Geometry: final body of the model. Coordinates: model frame, mm. A direction names the side the tool comes from. Give positions to 0.01 mm unless a question says otherwise; leave off trailing zeros. Loops run counter-clockwise (first coordinate to the right, second up) from the corner with the lowest first, then second, coordinate; pieces in that order, holes last. Notation, with made-up numbers: (-13.75, 0.25) -> (40.25, 0.25) arc R18 cw to (40.25, 17.25) -> close; hole circle Ø4 at (50.25, -21). An arc over 180 degrees is marked (long way). Answer in a Markdown table with one row per item. Add a question column.
from build123d import *

# Parameters (mm, degrees)
SKETCH1_W           = 80
SKETCH1_H           = 40
SKETCH1_R           = 1.5
SKETCH1_R_2         = 3
BOSS_EXTRUDE1_DEPTH = 4
EDGE_FLANGE1_DEPTH  = 40
SKETCH13_R          = 1.5
CUT_EXTRUDE1_DEPTH  = 4


# Sheet-metal steps are written as plain solids
with BuildPart() as part:
    # Sketch1 → Boss-Extrude1 (new body)
    with BuildSketch(Plane.XY):
        with Locations((10, 0)):
            Rectangle(SKETCH1_W, SKETCH1_H)
        with Locations((22, 12.5)):
            Circle(SKETCH1_R, mode=Mode.SUBTRACT)
        with Locations((-22, 12.5)):
            Circle(SKETCH1_R, mode=Mode.SUBTRACT)
        with Locations((-22, -12.5)):
            Circle(SKETCH1_R, mode=Mode.SUBTRACT)
        with Locations((22, -12.5)):
            Circle(SKETCH1_R, mode=Mode.SUBTRACT)
        with Locations((0, -1.5)):
            Circle(SKETCH1_R_2, mode=Mode.SUBTRACT)
    extrude(amount=BOSS_EXTRUDE1_DEPTH)

    # Edge-Flange1 section (across the edge) → Edge-Flange1 (add)
    with BuildSketch(Plane(origin=(55, 20, 0), x_dir=(-1, 0, 0), z_dir=(0, -1, 0))):
        with BuildLine():
            Line((-4, 5), (-4, 46))
            Line((-4, 46), (0, 46))
            Line((0, 46), (0, 5))
            ThreePointArc((0, 5), (1.464466094, 1.464466094), (5, 0))
            Line((5, 0), (5, -4))
            ThreePointArc((5, -4), (-1.363961031, -1.363961031), (-4, 5))
        make_face()
    extrude(amount=EDGE_FLANGE1_DEPTH)

    # Sketch13 → Cut-Extrude1 (cut)
    with BuildSketch(Plane.ZY.offset(-55)):
        with Locations((-38.5, 12.5)):
            Circle(SKETCH13_R)
        with Locations((-13.5, 12.5)):
            Circle(SKETCH13_R)
        with Locations((-13.5, -12.5)):
            Circle(SKETCH13_R)
        with Locations((-38.5, -12.5)):
            Circle(SKETCH13_R)
    extrude(amount=-CUT_EXTRUDE1_DEPTH, mode=Mode.SUBTRACT)


solid = part.part
(1) Cut plane A-A on z = -38.5. Return the cut outline in (x, y).
(2) Reachability of faces 1 (the flat face through (57, 0, -46)), 2 (the flat face through (9, 0, 0)) from +Z, -Z, +X, -X, +Y, -Y: full face, straight path, thin tool, end or side. Return the list, or none.
(3) Draft query along Y for faces 3 (the cylindrical face through (56.294, 0.28, 1.434)), 4 (the flat face through (27, -20, 1)), 5 (the cylindrical face through (56.97, -12.43, -15)), 6 (the cylindrical face through (-23.5, 12.57, 1.97)). Return one class per face: +Y half, -Y half, draft (parallel to the pull), parting line (faces both ways), or undercut.
(4) Cut plane B-B on x = 0. Return the cut outline in (y, z), then the cut area to 3 significant figures.
(5) Cut plane D-D on y = -9. Return the cut outline in (x, z), then the cut area to 3 significant figures.
(6) Pin query (flat end, axial travel): pin 1 Ø8 at (y, z) = (-9.5, -28) entering from -X; pin 2 Ø12 at (x, y) = (0, 4.5) entering from -Z; pin 3 Ø2.5 at (y, z) = (-12.5, -13.5) entering from -X. Return the tip coordinate at first contact, or that it passes through.
(7) Cut plane C-C on x = -22. Return the cut outline in (y, z).
(8) Material intervals for line 1 along Y through (x, z) = (-22, 0.9); line 2 along Y through (x, z) = (57, -38); line 3 along X through (y, z) = (12, 2), sorted ascending. Write a range as from..to.
Answer list:
| question | item | result |
|---|---|---|
| 1 | outline | (55, -20) -> (59, -20) -> (59, -14) -> (55, -14) -> close; (55, -11) -> (59, -11) -> (59, 11) -> (55, 11) -> close; (55, 14) -> (59, 14) -> (59, 20) -> (55, 20) -> close |
| 2 | face 1 | -Z, +X, -X, +Y, -Y |
| 2 | face 2 | -Z, -X, +Y, -Y |
| 3 | face 3 | draft |
| 3 | face 4 | -Y half |
| 3 | face 5 | undercut |
| 3 | face 6 | undercut |
| 4 | outline | (-20, 0) -> (-4.5, 0) -> (-4.5, 4) -> (-20, 4) -> close; (1.5, 0) -> (20, 0) -> (20, 4) -> (1.5, 4) -> close |
| 4 | area | 136 mm² |
| 5 | outline | (-30, 0) -> (50, 0) arc R5 cw to (55, -5) -> (55, -46) -> (59, -46) -> (59, -5) arc R9 ccw to (50, 4) -> (-30, 4) -> close |
| 5 | area | 528 mm² |
| 6 | pin 1 | stops at x = 55 |
| 6 | pin 2 | stops at z = 0 |
| 6 | pin 3 | passes through |
| 7 | outline | (-20, 0) -> (-14, 0) -> (-14, 4) -> (-20, 4) -> close; (-11, 0) -> (11, 0) -> (11, 4) -> (-11, 4) -> close; (14, 0) -> (20, 0) -> (20, 4) -> (14, 4) -> close |
| 8 | line 1 | y = -20..-14, -11..11, 14..20 |
| 8 | line 2 | y = -20..-13.91, -11.09..11.09, 13.91..20 |
| 8 | line 3 | x = -30..-23.41, -20.59..20.59, 23.41..55.66 |
